```python
from build123d import *

# Parameters (mm, degrees)
SKETCH009_W     = 98
SKETCH009_H     = 98
PAD003_DEPTH    = 3
SKETCH006_W     = 83.5
SKETCH006_H     = 83.5
PAD002_DEPTH    = 7
SKETCH011_R     = 39.5
POCKET007_DEPTH = 10
SKETCH007_W     = 80.5
SKETCH007_H     = 80.5
POCKET004_DEPTH = 2
SKETCH010_R     = 1.85
POCKET006_DEPTH = 8
SKETCH008_R     = 2.75
POCKET005_DEPTH = 5
CHAMFER001_SIZE = 0.5
SKETCH015_W     = 98
SKETCH015_H     = 98
PAD005_DEPTH    = 3
SKETCH012_W     = 83.5
SKETCH012_H     = 83.5
PAD004_DEPTH    = 7
SKETCH017_R     = 39.5
POCKET011_DEPTH = 10
SKETCH013_W     = 80.5
SKETCH013_H     = 80.5
POCKET008_DEPTH = 2
SKETCH016_R     = 1.85
POCKET010_DEPTH = 8
SKETCH014_R     = 2.75
POCKET009_DEPTH = 5
CHAMFER002_SIZE = 0.5
SKETCH021_W     = 98
SKETCH021_H     = 98
PAD007_DEPTH    = 3
SKETCH018_W     = 83.5
SKETCH018_H     = 83.5
PAD006_DEPTH    = 7
SKETCH023_R     = 39.5
POCKET015_DEPTH = 10
SKETCH019_W     = 80.5
SKETCH019_H     = 80.5
POCKET012_DEPTH = 2
SKETCH022_R     = 1.85
POCKET014_DEPTH = 8
SKETCH020_R     = 2.75
POCKET013_DEPTH = 5
CHAMFER003_SIZE = 0.5
SKETCH_W        = 98
SKETCH_H        = 98
PAD_DEPTH       = 3
SKETCH001_W     = 83.5
SKETCH001_H     = 83.5
PAD001_DEPTH    = 7
SKETCH002_R     = 39.5
POCKET_DEPTH    = 10
SKETCH003_W     = 80.5
SKETCH003_H     = 80.5
POCKET001_DEPTH = 2
SKETCH004_R     = 1.85
POCKET002_DEPTH = 8
SKETCH005_R     = 2.75
POCKET003_DEPTH = 5
CHAMFER_SIZE    = 0.5


with BuildPart() as body001:
    # Sketch009 → Pad003 (new body)
    with BuildSketch(Plane.XY):
        Rectangle(SKETCH009_W, SKETCH009_H)
    extrude(amount=PAD003_DEPTH)

    # Sketch006 (on Face6 of Pad003) → Pad002 (join)
    with BuildSketch(Plane.XY.offset(3)):
        Rectangle(SKETCH006_W, SKETCH006_H)
    extrude(amount=PAD002_DEPTH)

    # Sketch011 (on Face11 of Pad002) → Pocket007 (cut)
    with BuildSketch(Plane.XY.offset(10)):
        Circle(SKETCH011_R)
    extrude(amount=-POCKET007_DEPTH, mode=Mode.SUBTRACT)

    # Sketch007 (on Face12 of Pocket007) → Pocket004 (cut)
    with BuildSketch(Plane.XY.offset(10)):
        Rectangle(SKETCH007_W, SKETCH007_H)
    extrude(amount=-POCKET004_DEPTH, mode=Mode.SUBTRACT)

    # Sketch010 (on Face12 of Pocket004) → Pocket006 (cut)
    with BuildSketch(Plane.XY.offset(8)):
        with Locations((-35.75, 35.75)):
            Circle(SKETCH010_R)
        with Locations((35.75, 35.75)):
            Circle(SKETCH010_R)
        with Locations((35.75, -35.75)):
            Circle(SKETCH010_R)
        with Locations((-35.75, -35.75)):
            Circle(SKETCH010_R)
    extrude(amount=-POCKET006_DEPTH, mode=Mode.SUBTRACT)

    # Sketch008 (on Face4 of Pocket006) → Pocket005 (cut)
    with BuildSketch(Plane(origin=(0, 0, 0), x_dir=(1, 0, 0), z_dir=(0, 0, -1))):
        with Locations((-35.75, 35.75)):
            Circle(SKETCH008_R)
        with Locations((35.75, 35.75)):
            Circle(SKETCH008_R)
        with Locations((35.75, -35.75)):
            Circle(SKETCH008_R)
        with Locations((-35.75, -35.75)):
            Circle(SKETCH008_R)
    extrude(amount=-POCKET005_DEPTH, mode=Mode.SUBTRACT)

    # Chamfer001
    chamfer001_edges = [body001.edges().sort_by_distance(p)[0] for p in [
        (33, 35.75, 0),
        (33, -35.75, 0),
        (-38.5, -35.75, 0),
        (-38.5, 35.75, 0),
    ]]
    chamfer(chamfer001_edges, length=CHAMFER001_SIZE)


with BuildPart() as body001_1:
    # Body001 placement: moved
    add(body001.part.moved(Location((98, 0, 0))))


with BuildPart() as body002:
    # Sketch015 → Pad005 (new body)
    with BuildSketch(Plane.XY):
        Rectangle(SKETCH015_W, SKETCH015_H)
    extrude(amount=PAD005_DEPTH)

    # Sketch012 (on Face6 of Pad005) → Pad004 (join)
    with BuildSketch(Plane.XY.offset(3)):
        Rectangle(SKETCH012_W, SKETCH012_H)
    extrude(amount=PAD004_DEPTH)

    # Sketch017 (on Face11 of Pad004) → Pocket011 (cut)
    with BuildSketch(Plane.XY.offset(10)):
        Circle(SKETCH017_R)
    extrude(amount=-POCKET011_DEPTH, mode=Mode.SUBTRACT)

    # Sketch013 (on Face12 of Pocket011) → Pocket008 (cut)
    with BuildSketch(Plane.XY.offset(10)):
        Rectangle(SKETCH013_W, SKETCH013_H)
    extrude(amount=-POCKET008_DEPTH, mode=Mode.SUBTRACT)

    # Sketch016 (on Face12 of Pocket008) → Pocket010 (cut)
    with BuildSketch(Plane.XY.offset(8)):
        with Locations((-35.75, 35.75)):
            Circle(SKETCH016_R)
        with Locations((35.75, 35.75)):
            Circle(SKETCH016_R)
        with Locations((35.75, -35.75)):
            Circle(SKETCH016_R)
        with Locations((-35.75, -35.75)):
            Circle(SKETCH016_R)
    extrude(amount=-POCKET010_DEPTH, mode=Mode.SUBTRACT)

    # Sketch014 (on Face4 of Pocket010) → Pocket009 (cut)
    with BuildSketch(Plane(origin=(0, 0, 0), x_dir=(1, 0, 0), z_dir=(0, 0, -1))):
        with Locations((-35.75, 35.75)):
            Circle(SKETCH014_R)
        with Locations((35.75, 35.75)):
            Circle(SKETCH014_R)
        with Locations((35.75, -35.75)):
            Circle(SKETCH014_R)
        with Locations((-35.75, -35.75)):
            Circle(SKETCH014_R)
    extrude(amount=-POCKET009_DEPTH, mode=Mode.SUBTRACT)

    # Chamfer002
    chamfer002_edges = [body002.edges().sort_by_distance(p)[0] for p in [
        (33, 35.75, 0),
        (33, -35.75, 0),
        (-38.5, -35.75, 0),
        (-38.5, 35.75, 0),
    ]]
    chamfer(chamfer002_edges, length=CHAMFER002_SIZE)


with BuildPart() as body002_1:
    # Body002 placement: moved
    add(body002.part.moved(Location((0, 98, 0))))


with BuildPart() as body003:
    # Sketch021 → Pad007 (new body)
    with BuildSketch(Plane.XY):
        Rectangle(SKETCH021_W, SKETCH021_H)
    extrude(amount=PAD007_DEPTH)

    # Sketch018 (on Face6 of Pad007) → Pad006 (join)
    with BuildSketch(Plane.XY.offset(3)):
        Rectangle(SKETCH018_W, SKETCH018_H)
    extrude(amount=PAD006_DEPTH)

    # Sketch023 (on Face11 of Pad006) → Pocket015 (cut)
    with BuildSketch(Plane.XY.offset(10)):
        Circle(SKETCH023_R)
    extrude(amount=-POCKET015_DEPTH, mode=Mode.SUBTRACT)

    # Sketch019 (on Face12 of Pocket015) → Pocket012 (cut)
    with BuildSketch(Plane.XY.offset(10)):
        Rectangle(SKETCH019_W, SKETCH019_H)
    extrude(amount=-POCKET012_DEPTH, mode=Mode.SUBTRACT)

    # Sketch022 (on Face12 of Pocket012) → Pocket014 (cut)
    with BuildSketch(Plane.XY.offset(8)):
        with Locations((-35.75, 35.75)):
            Circle(SKETCH022_R)
        with Locations((35.75, 35.75)):
            Circle(SKETCH022_R)
        with Locations((35.75, -35.75)):
            Circle(SKETCH022_R)
        with Locations((-35.75, -35.75)):
            Circle(SKETCH022_R)
    extrude(amount=-POCKET014_DEPTH, mode=Mode.SUBTRACT)

    # Sketch020 (on Face4 of Pocket014) → Pocket013 (cut)
    with BuildSketch(Plane(origin=(0, 0, 0), x_dir=(1, 0, 0), z_dir=(0, 0, -1))):
        with Locations((-35.75, 35.75)):
            Circle(SKETCH020_R)
        with Locations((35.75, 35.75)):
            Circle(SKETCH020_R)
        with Locations((35.75, -35.75)):
            Circle(SKETCH020_R)
        with Locations((-35.75, -35.75)):
            Circle(SKETCH020_R)
    extrude(amount=-POCKET013_DEPTH, mode=Mode.SUBTRACT)

    # Chamfer003
    chamfer003_edges = [body003.edges().sort_by_distance(p)[0] for p in [
        (33, 35.75, 0),
        (33, -35.75, 0),
        (-38.5, -35.75, 0),
        (-38.5, 35.75, 0),
    ]]
    chamfer(chamfer003_edges, length=CHAMFER003_SIZE)


with BuildPart() as body003_1:
    # Body003 placement: moved
    add(body003.part.moved(Location((98, 98, 0))))


with BuildPart() as body004:
    # Sketch → Pad (new body)
    with BuildSketch(Plane.XY):
        Rectangle(SKETCH_W, SKETCH_H)
    extrude(amount=PAD_DEPTH)

    # Sketch001 (on Face6 of Pad) → Pad001 (join)
    with BuildSketch(Plane.XY.offset(3)):
        Rectangle(SKETCH001_W, SKETCH001_H)
    extrude(amount=PAD001_DEPTH)

    # Sketch002 (on Face11 of Pad001) → Pocket (cut)
    with BuildSketch(Plane.XY.offset(10)):
        Circle(SKETCH002_R)
    extrude(amount=-POCKET_DEPTH, mode=Mode.SUBTRACT)

    # Sketch003 (on Face12 of Pocket) → Pocket001 (cut)
    with BuildSketch(Plane.XY.offset(10)):
        Rectangle(SKETCH003_W, SKETCH003_H)
    extrude(amount=-POCKET001_DEPTH, mode=Mode.SUBTRACT)

    # Sketch004 (on Face12 of Pocket001) → Pocket002 (cut)
    with BuildSketch(Plane.XY.offset(8)):
        with Locations((-35.75, 35.75)):
            Circle(SKETCH004_R)
        with Locations((35.75, 35.75)):
            Circle(SKETCH004_R)
        with Locations((35.75, -35.75)):
            Circle(SKETCH004_R)
        with Locations((-35.75, -35.75)):
            Circle(SKETCH004_R)
    extrude(amount=-POCKET002_DEPTH, mode=Mode.SUBTRACT)

    # Sketch005 (on Face4 of Pocket002) → Pocket003 (cut)
    with BuildSketch(Plane(origin=(0, 0, 0), x_dir=(1, 0, 0), z_dir=(0, 0, -1))):
        with Locations((-35.75, 35.75)):
            Circle(SKETCH005_R)
        with Locations((35.75, 35.75)):
            Circle(SKETCH005_R)
        with Locations((35.75, -35.75)):
            Circle(SKETCH005_R)
        with Locations((-35.75, -35.75)):
            Circle(SKETCH005_R)
    extrude(amount=-POCKET003_DEPTH, mode=Mode.SUBTRACT)

    # Chamfer
    chamfer_edges = [body004.edges().sort_by_distance(p)[0] for p in [
        (33, 35.75, 0),
        (33, -35.75, 0),
        (-38.5, -35.75, 0),
        (-38.5, 35.75, 0),
    ]]
    chamfer(chamfer_edges, length=CHAMFER_SIZE)

    # Fusion: union Body001, Body002, Body003
    add(body001_1.part)
    add(body002_1.part)
    add(body003_1.part)


solid = body004.part
```
Check sheet for the modelled part. Datum: model origin and axes. Units: mm. A direction names the side the tool comes from. Round coordinates to 2 decimals unless told otherwise and drop trailing zeros. Write each loop counter-clockwise with the first axis right and the second up, starting at its lowest first coordinate (ties: lowest second). Pieces come first, ordered by that corner, then holes. Notation, with made-up numbers: M -13,8 L 4,8 A24 cw 4,31 Z; hole C 56.5,-36.75 d5. An arc over 180 degrees is marked long. Write item = value, one per line. Start each with the question number.
1. Scan lines: line 1 (Y direction, x = 116, z = 9.25); line 2 (X direction, y = 1.5, z = 7.25); line 3 (X direction, y = 66, z = 2.25). Record each from-to range of solid material in increasing order. Write a range as [from, to].
2. Gauge pin test, flat ends, axial feed: pin 1 (5 mm diameter, centred on x = -27.5, y = 60.5, fed in from +Z); pin 2 (2 mm diameter, centred on x = 35.75, y = 133.75, fed in from +Z); pin 3 (4.5 mm diameter, centred on x = 36, y = 133.5, fed in from -Z); pin 4 (1 mm diameter, centred on x = 101, z = 9, fed in from +Y). Record the tip position at first contact, or that the pin passes through.
3. Tool access check on faces 1 (the flat face through (38, -35, 5)), 2 (the flat face through (-18.8, 138.4, 10)), 3 (the flat face through (-1, 56.25, 6)), 4 (the flat face through (89, -39, 8)), 5 (the flat face through (-41.75, -1, 6)). Record the directions out of +Z, -Z, +X, -X, +Y, -Y that give a thin tool (end or side, any length) a straight path to the whole face; none if there is none.
4. Release check for a two-part mould opening along Y. For faces 6 (the flat face through (136, 63, 5)), 7 (the flat face through (-41.75, 97, 6)) record: pulls with the +Y half, pulls with the -Y half, needs draft (parallel to the pull), parting line crosses it, or undercut.
5. Section check A-A, the plane x = 0. Record the cut outline in (y, z), then the cut area to 3 significant figures.
6. Section check B-B, the plane y = 127.5. Record the cut outline in (x, z).
Results found:
q1.line_1 = [-41.75, -40.25], [40.25, 41.75], [56.25, 57.75], [138.25, 139.75]
q1.line_2 = [-41.75, -39.47], [39.47, 41.75], [56.25, 58.53], [137.47, 139.75]
q1.line_3 = [-49, -23.16], [23.16, 74.84], [121.16, 147]
q2.pin_1 = 8
q2.pin_2 = through
q2.pin_3 = 5
q2.pin_4 = 139.75
q3.face_1 = -Z
q3.face_2 = +Z, +X, -X, +Y, -Y
q3.face_3 = +Z, +X, -X
q3.face_4 = +Z
q3.face_5 = +Z, -X, +Y, -Y
q4.face_6 = undercut
q4.face_7 = needs draft
q5.outline = M -49,0 L -39.5,0 L -39.5,8 L -40.25,8 L -40.25,10 L -41.75,10 L -41.75,3 L -49,3 Z; M 39.5,0 L 58.5,0 L 58.5,8 L 57.75,8 L 57.75,10 L 56.25,10 L 56.25,3 L 41.75,3 L 41.75,10 L 40.25,10 L 40.25,8 L 39.5,8 Z; M 137.5,0 L 147,0 L 147,3 L 139.75,3 L 139.75,10 L 138.25,10 L 138.25,8 L 137.5,8 Z
q5.area = 171 mm^2
q6.outline = M -49,0 L -26.27,0 L -26.27,8 L -40.25,8 L -40.25,10 L -41.75,10 L -41.75,3 L -49,3 Z; M 26.27,0 L 71.73,0 L 71.73,8 L 57.75,8 L 57.75,10 L 56.25,10 L 56.25,3 L 41.75,3 L 41.75,10 L 40.25,10 L 40.25,8 L 26.27,8 Z; M 124.27,0 L 147,0 L 147,3 L 139.75,3 L 139.75,10 L 138.25,10 L 138.25,8 L 124.27,8 Z
